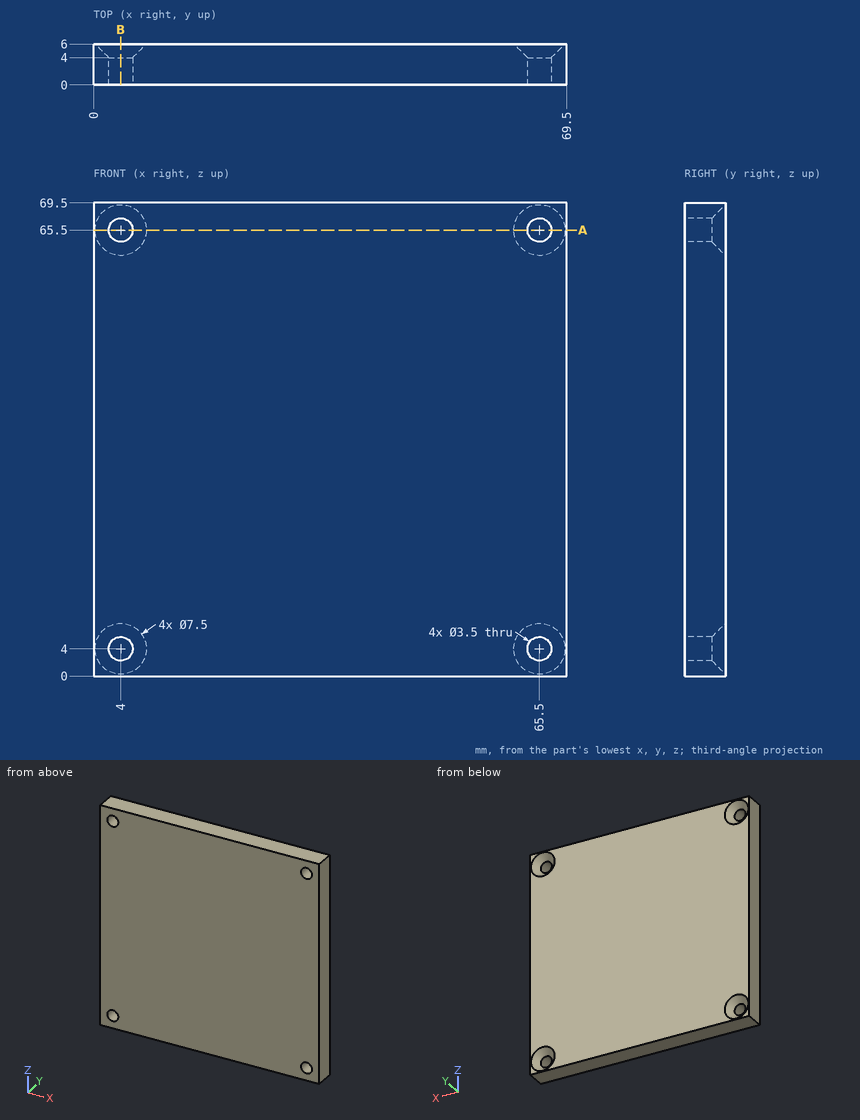
Can you work these out from the drawing? Everything is in mm from the part's minimum corner. Round coordinates to 2 decimals unless told otherwise and drop trailing zeros. Order: outer loops, then holes, each group sorted by start corner. A loop starts at its lowest first (then second) coordinate and runs counter-clockwise, first axis right, second up. Notation, with made-up numbers: M 80,89 L 124,89 A15 cw 124,95 Z; hole C 66,54 d8. An arc over 180 degrees is marked long. Answer as CSV lines item,"result".
Item 1: Imagine slicing it at A-A on z = 65.5. List the corners of the cut face in (x, y) for me, and give its area (3 significant figures).
From the geometry:
outline,"M 0,0 L 2.25,0 L 2.25,4 L 0.25,6 L 0,6 Z; M 5.75,0 L 63.75,0 L 63.75,4 L 61.75,6 L 7.75,6 L 5.75,4 Z; M 67.25,0 L 69.5,0 L 69.5,6 L 69.25,6 L 67.25,4 Z"
area,"367 mm2"
Item 2: Imagine slicing it at B-B on x = 4. List the corners of the cut face in (y, z) for me.
From the geometry:
outline,"M 0,0 L 6,0 L 6,0.25 L 4,2.25 L 0,2.25 Z; M 0,5.75 L 4,5.75 L 6,7.75 L 6,61.75 L 4,63.75 L 0,63.75 Z; M 0,67.25 L 4,67.25 L 6,69.25 L 6,69.5 L 0,69.5 Z"
Item 3: Please list where this line runs through material, in increasing order: L1, parallel to Z at x = 65.5, y = 1.7. Write a range as [from, to].
From the geometry:
L1,"[0, 2.25], [5.75, 63.75], [67.25, 69.5]"
Item 4: For pin 1 (2 mm diameter, centred on x = 65.5, z = 4, fed in from +Y), with a flat end and sliding along its axis, tell me the tip position at first contact or that it passes through.
From the geometry:
pin 1,"through"
